Verification items for the finished model (mm, model axes). A direction names the side the tool comes from. Coordinates: 2 decimals unless noted, no trailing zeros. Loops run counter-clockwise (first coordinate to the right, second up) from the corner with the lowest first, then second, coordinate; pieces in that order, holes last. Notation, with made-up numbers: (44.25, 3.25) - (97.25, 3.25) arc R29 cw to (97.25, 32.25) - close; hole circle Ø9 at (-8, -25). An arc over 180 degrees is marked (long way). One line per item, written item: value. Start each with the question number.
(1) Gauge pin test, flat end, axial feed: P1, Ø5, axis at x = 10, z = -7, coming from the +Y side. Record the tip position at first contact, or that the pin passes through.
(2) Section check A-A (y = 1.1). Record the boundary of the cut face in (x, z) (3 decimals), plus the area to 3 significant figures.
(3) Section check C-C (z = -1). Record the boundary of the cut face in (x, y) (3 decimals).
(4) Set-up check for faces 5 (the face through (6, 0, -6)), 6 (the face through (0.635, 1, -6)): record each of +Z, -Z, +X, -X, +Y, -Y from which the full face is reachable in a straight line by a thin tool's end or side.
(5) Draft check along Z on faces 1 (the face through (6, 1, -12.7)), 2 (the face through (8.83, 0.97, -6.9)), 3 (the face through (5, 1.905, -9)), 4 (the face through (0, 1, -6)). Enter one of: +Z half, -Z half, draft (parallel to the pull), parting line (faces both ways), or undercut.
(6) Thickness scan on probe 1 along Z at (x, y) = (6.25, 1.3) (3 decimals); probe 2 along X at (y, z) = (0.5, -10.5) (3 decimals); probe 3 along Z at (x, y) = (10.5, 1.25) (3 decimals). Record the ranges inside material, lowest first. Write a range as [from, to].
(7) Section check D-D (z = -6.35). Record the boundary of the cut face in (x, y) (3 decimals), plus the area to 3 significant figures.
```python
from build123d import *

# Parameters (mm, degrees)
SKETCH1_W           = 12.7
SKETCH1_H           = 12.7
BOSS_EXTRUDE1_DEPTH = 2.54
FILLET1_R           = 0.635
SHELL1_START        = 0.635
SHELL1_OUTLINE_W    = 1.905
SHELL1_OUTLINE_H    = 11.43
SHELL1_DEPTH        = 11.43
SKETCH2_R           = 2.54
BOSS_EXTRUDE2_DEPTH = 1.905
SKETCH4_W           = 1.099038461
SKETCH4_H           = 0.529166666
SKETCH4_W_2         = 2.238782051
SKETCH4_H_2         = 0.203525641
BOSS_EXTRUDE4_DEPTH = 0.00254


# Read off the part's stored shape, not the designer's step: Shell1
with BuildPart() as part:
    # Sketch1 → Boss-Extrude1 (new body)
    with BuildSketch(Plane(origin=(0, 0, 0), x_dir=(1, 0, 0), z_dir=(0, 1, 0))):
        with Locations((6.35, 6.35)):
            Rectangle(SKETCH1_W, SKETCH1_H)
    extrude(amount=BOSS_EXTRUDE1_DEPTH)

    # Fillet1
    fillet1_edges = [part.edges().sort_by_distance(p)[0] for p in [
        (0, 1.27, -12.7),
        (12.7, 1.27, -12.7),
        (12.7, 1.27, 0),
        (0, 1.27, 0),
    ]]
    fillet(fillet1_edges, radius=FILLET1_R)

    # Shell1 outline → Shell1 (cut)
    with BuildSketch(Plane.YZ.offset(SHELL1_START)):
        with Locations((0.9525, -6.35)):
            Rectangle(SHELL1_OUTLINE_W, SHELL1_OUTLINE_H)
    extrude(amount=SHELL1_DEPTH, mode=Mode.SUBTRACT)

    # Sketch2 → Boss-Extrude2 (add)
    with BuildSketch(Plane(origin=(0, 1.905, 0), x_dir=(-1, 0, 0), z_dir=(0, -1, 0))):
        with Locations(Location((-6.35, 6.35, 0), (0, 0, 270))):
            Circle(SKETCH2_R)
    extrude(amount=BOSS_EXTRUDE2_DEPTH)

    # Sketch4 → Boss-Extrude4 (add)
    with BuildSketch(Plane(origin=(0, 2.54, 0), x_dir=(1, 0, 0), z_dir=(0, 1, 0))):
        with Locations((6.173665384, 3.700096154)):
            Rectangle(SKETCH4_W, SKETCH4_H)
        with Locations((6.199391026, 7.913891026)):
            Rectangle(SKETCH4_W_2, SKETCH4_H_2)
    extrude(amount=BOSS_EXTRUDE4_DEPTH)


solid = part.part
```
Responses:
1. P1: stops at y = 2.54
2. outline: (0, -12.065) arc R0.635 ccw to (0.635, -12.7) - (12.065, -12.7) arc R0.635 ccw to (12.7, -12.065) - (12.7, -0.635) arc R0.635 ccw to (12.065, 0) - (0.635, 0) arc R0.635 ccw to (0, -0.635) - close; circle Ø5.08 at (6.35, -6.35); hole (0.635, -12.065) - (12.065, -12.065) - (12.065, -0.635) - (0.635, -0.635) - close
2. area: 50.6 mm²
3. outline: (0, 0) - (0.635, 0) - (0.635, 1.905) - (12.065, 1.905) - (12.065, 0) - (12.7, 0) - (12.7, 2.54) - (0, 2.54) - close
4. face 5: +Z, -Z, +X, -X, -Y
4. face 6: -Y
5. face 1: -Z half
5. face 2: undercut
5. face 3: undercut
5. face 4: draft
6. probe 1: z = [-12.7, -12.065], [-8.888, -3.812], [-0.635, 0]
6. probe 2: x = [0, 0.635], [12.065, 12.7]
6. probe 3: z = [-12.7, -12.065], [-0.635, 0]
7. outline: (0, 0) - (0.635, 0) - (0.635, 1.905) - (3.81, 1.905) - (3.81, 0) - (8.89, 0) - (8.89, 1.905) - (12.065, 1.905) - (12.065, 0) - (12.7, 0) - (12.7, 2.54) - (0, 2.54) - close
7. area: 20.2 mm²
